The listing builds one solid part. Answer for the finished solid, in the listing's coordinates (mm). A direction names the side the tool comes from. Give positions to 0.01 mm unless a question says otherwise; leave off trailing zeros. Write each loop counter-clockwise with the first axis right and the second up, starting at its lowest first coordinate (ties: lowest second). Pieces come first, ordered by that corner, then holes. Notation, with made-up numbers: (-4.5, -6) - (43.5, -6) arc R15 ccw to (43.5, 9) - close; hole circle Ø6 at (28, -21). An arc over 180 degrees is marked (long way). Return JSON: item names as keys, results as strings.
Autodesk Inventor part; units mm, degrees
ref_plane "YZ Plane" through (0, 0, 0) normal (1, 0, 0) x (0, 1, 0)
ref_plane "XZ Plane" through (0, 0, 0) normal (0, 1, 0) x (-1, 0, 0)
ref_plane "XY Plane" through (0, 0, 0) normal (0, 0, 1) x (1, 0, 0)
sketch "Sketch1" plane through (0, 0, 0) normal (0, 0, 1) x (1, 0, 0)
  line L0 (-110.675, 126.35) -> (-171, 126.35)
  line L1 (-171, 126.35) -> (-171, 59.04)
  line L2 (-171, 59.04) -> (-110.675, 59.04)
  line L3 (-110.675, 59.04) -> (-110.675, 126.35)
  point P0 (0, 0)
  dimension "d0" = 60.325
  dimension "d1" = 67.31
extrude "Extrusion1" add sketch "Sketch1" along normal blind 3.175
sketch "Sketch2" plane through (0, 0, 3.175) normal (0, 0, 1) x (1, 0, 0)
  line L0 (-171, 126.35) -> (-171, 59.04)
  line L1 (-171, 59.04) -> (-167.825, 59.04)
  line L2 (-167.825, 59.04) -> (-167.825, 74.915)
  line L3 (-167.825, 74.915) -> (-171, 74.915)
  line L4 (-171, 74.915) -> (-171, 59.04)
  line L5 (-171, 85.075) -> (-167.825, 85.075)
  line L6 (-167.825, 85.075) -> (-167.825, 100.315)
  line L7 (-167.825, 100.315) -> (-171, 100.315)
  line L8 (-171, 100.315) -> (-171, 85.075)
  line L9 (-110.675, 126.35) -> (-171, 126.35)
  line L10 (-171, 126.35) -> (-167.825, 126.35)
  line L11 (-167.825, 126.35) -> (-167.825, 110.475)
  line L12 (-167.825, 110.475) -> (-171, 110.475)
  line L13 (-171, 110.475) -> (-171, 126.35)
  point P0 (0, 0)
  dimension "d4" = 3.175
  dimension "d5" = 15.875
  dimension "d6" = 10.16
  dimension "d7" = 15.875
  dimension "d8" = 10.16
extrude "Extrusion3" cut sketch "Sketch2" against normal blind 3.175
ref_plane "Work Plane1" through (-140.8375, 59.04, 0) normal (1, 0, 0) x (0, 0, -1)
mirror "Mirror1" about plane through (-140.8375, 59.04, 0) normal (1, 0, 0) of "Extrusion3"
sketch "Sketch3" plane through (0, 0, 3.175) normal (0, 0, 1) x (1, 0, 0)
  line L0 (-123.375, 59.04) -> (-110.675, 59.04)
  line L1 (-110.675, 59.04) -> (-110.675, 62.215)
  line L2 (-110.675, 62.215) -> (-123.375, 62.215)
  line L3 (-123.375, 62.215) -> (-123.375, 59.04)
  line L4 (-167.825, 59.04) -> (-113.85, 59.04)
  line L5 (-110.675, 74.915) -> (-110.675, 85.075)
  line L6 (-140.8375, 59.04) -> (-132.265, 59.04)
  line L7 (-132.265, 59.04) -> (-132.265, 62.215)
  line L8 (-132.265, 62.215) -> (-140.8375, 62.215)
  line L9 (-140.8375, 62.215) -> (-140.8375, 59.04)
  point P0 (0, 0)
  dimension "d13" = 12.7
  dimension "d14" = 3.175
  dimension "d15" = 8.89
extrude "Extrusion4" cut sketch "Sketch3" against normal blind 3.175
mirror "Mirror2" about plane through (-140.8375, 59.04, 0) normal (1, 0, 0) of "Extrusion4"
ref_plane "Work Plane2" through (-158.3, 92.695, 0) normal (0, -1, 0) x (1, 0, 0)
mirror "Mirror3" about plane through (-158.3, 92.695, 0) normal (0, -1, 0) of "Extrusion4", "Mirror2"
sketch "Sketch4" plane through (0, 0, 0) normal (0, 0, -1) x (-1, 0, 0)
  line L0 (149.41, 123.175) -> (132.265, 123.175)
  line L1 (148.14, 123.175) -> (133.916, 123.175)
  line L2 (133.916, 123.175) -> (133.916, 105.395)
  line L3 (133.916, 105.395) -> (148.14, 105.395)
  line L4 (148.14, 105.395) -> (148.14, 123.175)
  line L5 (110.675, 100.315) -> (110.675, 110.475)
  line L6 (171, 110.475) -> (171, 100.315)
  point P0 (0, 0)
  dimension "d18" = 17.78
  dimension "d19" = 14.224
  dimension "d21" = 22.86
extrude "Extrusion5" cut sketch "Sketch4" against normal blind 3.175
sketch "Sketch5" plane through (0, 0, 0) normal (0, 0, -1) x (-1, 0, 0)
  line L0 (153.5375, 68.565) -> (128.1375, 68.565)
  line L1 (128.1375, 68.565) -> (128.1375, 93.965)
  line L2 (128.1375, 93.965) -> (153.5375, 93.965)
  line L3 (153.5375, 93.965) -> (153.5375, 68.565)
  line L4 (140.8375, -25.27) -> (140.8375, 151.62)
  line L5 (132.265, 62.215) -> (149.41, 62.215)
  line L6 (145.6, 68.565) -> (136.075, 68.565)
  line L7 (136.075, 68.565) -> (136.075, 71.74)
  line L8 (136.075, 71.74) -> (145.6, 71.74)
  line L9 (145.6, 71.74) -> (145.6, 68.565)
  line L10 (145.6, 93.965) -> (136.075, 93.965)
  line L11 (136.075, 93.965) -> (136.075, 90.79)
  line L12 (136.075, 90.79) -> (145.6, 90.79)
  line L13 (145.6, 90.79) -> (145.6, 93.965)
  line L14 (153.5375, 76.5025) -> (150.3625, 76.5025)
  line L15 (150.3625, 76.5025) -> (150.3625, 86.0275)
  line L16 (150.3625, 86.0275) -> (153.5375, 86.0275)
  line L17 (153.5375, 86.0275) -> (153.5375, 76.5025)
  line L18 (128.1375, 86.0275) -> (131.3125, 86.0275)
  line L19 (131.3125, 86.0275) -> (131.3125, 76.5025)
  line L20 (131.3125, 76.5025) -> (128.1375, 76.5025)
  line L21 (128.1375, 76.5025) -> (128.1375, 86.0275)
  point P0 (0, 0)
  dimension "d24" = 25.4
  dimension "d25" = 25.4
  dimension "d26" = 12.7
  dimension "d27" = 6.35
  dimension "d28" = 3.175
  dimension "d29" = 7.9375
  dimension "d30" = 7.9375
  dimension "d31" = 3.175
  dimension "d32" = 7.9375
  dimension "d33" = 3.175
  dimension "d34" = 7.9375
  dimension "d35" = 3.175
extrude "Extrusion6" cut sketch "Sketch5" against normal blind 3.175 contours L0 L4 L8 L9 | L14 L15 L16 L3 | L0 L7 L8 L4 | L12 L11 L2 L4 | L4 L2 L13 L12 | L1 L18 L19 L20
Item 1: Flat-ended cylindrical pins translate along their axes: P1, Ø1.6, axis at x = -142, z = 1.5, coming from the -Y side (3 decimals); P2, Ø1, axis at y = 71, z = 1.5, coming from the -X side (3 decimals); P3, Ø1, axis at y = 124.5, z = 1.5, coming from the +X side (3 decimals). Find the tip coordinate at first contact, or state that the pin passes through.
Answer below:
{"P1": "stops at y = 62.215", "P2": "stops at x = -167.825", "P3": "stops at x = -123.375"}
Item 2: A cutting plane is placed at D-D on x = -163.5. Determine the outline of the cut face in (y, z) (3 decimals).
Answer below:
{"outline": "(62.215, 0) - (123.175, 0) - (123.175, 3.175) - (62.215, 3.175) - close"}
Item 3: For faces 1 (the face through (-112, 110.475, 2)), 2 (the face through (-163, 123.175, 2)), 3 (the face through (-145.6, 70, 2)), 4 (the face through (-112, 74.915, 2)), determine the directions among +Z, -Z, +X, -X, +Y, -Y from which every point of the face is accessible in a straight line to the end or side of a thin tool.
Answer below:
{"face 1": "+Z, -Z, +X, +Y", "face 2": "+Z, -Z, -X, +Y", "face 3": "+Z, -Z", "face 4": "+Z, -Z, +X, -Y"}
Item 4: A cutting plane is placed at A-A on y = 115. Determine the outline of the cut face in (x, z) (3 decimals), then the cut area to 3 significant figures.
Answer below:
{"outline": "(-167.825, 0) - (-148.14, 0) - (-148.14, 3.175) - (-167.825, 3.175) - close; (-133.916, 0) - (-113.85, 0) - (-113.85, 3.175) - (-133.916, 3.175) - close", "area": "126 mm²"}
Item 5: A cutting plane is placed at C-C on z = 1.6. Give the number of separate pieces and of enclosed holes in the cut face, then the cut area to 3 significant figures.
Answer below:
{"separate pieces": "1", "enclosed holes": "4", "area": "3,160 mm²"}
Item 6: The mould has two halves that part along Y. Classify faces 5 (the face through (-113.85, 117, 2)), 6 (the face through (-119, 62.215, 2)), 7 (the face through (-112, 100.315, 2)): +Y half, -Y half, draft (parallel to the pull), parting line (faces both ways), or undercut.
Answer below:
{"face 5": "draft", "face 6": "-Y half", "face 7": "undercut"}
Item 7: Consider L1, parallel to Y at x = -136.5, z = 3 (3 decimals); L2, parallel to X at y = 83, z = 1.5 (1 decimal); L3, parallel to Y at x = -129.5, z = 2.25. Determine where each line is inside the solid, lowest interval first.
Answer below:
{"L1": "y = 62.215 to 68.565, 71.74 to 90.79, 93.965 to 105.395", "L2": "x = -171 to -153.5, -150.4 to -131.3, -128.1 to -110.7", "L3": "y = 59.04 to 76.5, 86.03 to 126.35"}
Item 8: A cutting plane is placed at B-B on x = -138.5. Determine the outline of the cut face in (y, z) (3 decimals), then the cut area to 3 significant figures.
Answer below:
{"outline": "(62.215, 0) - (68.565, 0) - (68.565, 3.175) - (62.215, 3.175) - close; (71.74, 0) - (90.79, 0) - (90.79, 3.175) - (71.74, 3.175) - close; (93.965, 0) - (105.395, 0) - (105.395, 3.175) - (93.965, 3.175) - close", "area": "117 mm²"}
